```python
from build123d import *

# Parameters (mm, degrees)
F0_W           = 42.3
F0_H           = 42.3
F0_R           = 12
F0_R_2         = 2.5
F0_H_2         = 2
F1_DEPTH       = 5
F2_DEPTH       = 30
F5_D           = 5
F5_DEPTH       = 12.7
F5_TIP         = 1.5021515476
F5_ON_F4_D     = 5
F5_ON_F4_DEPTH = 12.7
F5_ON_F4_TIP   = 1.5021515476


with BuildPart() as f1:
    # F0 (on Top) → F1 (new body)
    with BuildSketch(Plane.XY):
        Polygon((-21.15, 21.15), (21.15, 21.15), (23.15, 21.15), (23.15, 23.15), (-23.15, 23.15), (-23.15, 21.15), align=None)
        Rectangle(F0_W, F0_H)
        with BuildLine():
            ThreePointArc((-15.5, 13.8), (-16.702081528, 16.702081528), (-13.8, 15.5))
            Line((-13.8, 15.5), (13.8, 15.5))
            ThreePointArc((13.8, 15.5), (15.5, 17.2), (17.2, 15.5))
            ThreePointArc((17.2, 15.5), (16.702081528, 14.297918472), (15.5, 13.8))
            Line((15.5, 13.8), (15.5, -13.8))
            ThreePointArc((15.5, -13.8), (16.702081528, -14.297918472), (17.2, -15.5))
            ThreePointArc((17.2, -15.5), (15.5, -17.2), (13.8, -15.5))
            Line((13.8, -15.5), (-13.8, -15.5))
            ThreePointArc((-13.8, -15.5), (-16.702081528, -16.702081528), (-15.5, -13.8))
            Line((-15.5, -13.8), (-15.5, 13.8))
        make_face(mode=Mode.SUBTRACT)
        with BuildLine():
            Line((13.8, 15.5), (-13.8, 15.5))
            ThreePointArc((-13.8, 15.5), (-14.297918472, 14.297918472), (-15.5, 13.8))
            Line((-15.5, 13.8), (-15.5, -13.8))
            ThreePointArc((-15.5, -13.8), (-14.297918472, -14.297918472), (-13.8, -15.5))
            Line((-13.8, -15.5), (13.8, -15.5))
            ThreePointArc((13.8, -15.5), (14.297918472, -14.297918472), (15.5, -13.8))
            Line((15.5, -13.8), (15.5, 13.8))
            ThreePointArc((15.5, 13.8), (14.297918472, 14.297918472), (13.8, 15.5))
        make_face()
        Circle(F0_R, mode=Mode.SUBTRACT)
        Polygon((23.15, 23.15), (23.15, 21.15), (23.15, -23.15), (53.15, -23.15), (53.15, 53.15), (-53.15, 53.15), (-53.15, -23.15), (-23.15, -23.15), (-23.15, 21.15), (-23.15, 23.15), align=None)
        with Locations((-38.15, -8.15)):
            Circle(F0_R_2, mode=Mode.SUBTRACT)
        with Locations((38.15, -8.15)):
            Circle(F0_R_2, mode=Mode.SUBTRACT)
        with Locations((-38.15, 38.15)):
            Circle(F0_R_2, mode=Mode.SUBTRACT)
        with Locations((38.15, 38.15)):
            Circle(F0_R_2, mode=Mode.SUBTRACT)
        Polygon((-21.15, -21.15), (-21.15, 21.15), (-23.15, 21.15), (-23.15, -23.15), (-21.15, -23.15), align=None)
        Polygon((23.15, 21.15), (21.15, 21.15), (21.15, -21.15), (21.15, -23.15), (23.15, -23.15), align=None)
        with Locations((0, -22.15)):
            Rectangle(F0_W, F0_H_2)
    extrude(amount=F1_DEPTH)

    # F0 (on Top) → F2 (join)
    with BuildSketch(Plane.XY):
        Polygon((-21.15, 21.15), (21.15, 21.15), (23.15, 21.15), (23.15, 23.15), (-23.15, 23.15), (-23.15, 21.15), align=None)
        Polygon((23.15, 21.15), (21.15, 21.15), (21.15, -21.15), (21.15, -23.15), (23.15, -23.15), align=None)
    extrude(amount=-F2_DEPTH)

    # F5
    with Locations(Plane.XZ.offset(-21.15)):
        with Locations((0, -15)):
            Hole(F5_D / 2, depth=F5_DEPTH)
            with Locations((0, 0, -(F5_DEPTH + F5_TIP / 2))):  # 118° drill point
                Cone(0, F5_D / 2, F5_TIP, mode=Mode.SUBTRACT)

    # F5 on F4
    with Locations(Plane(origin=(21.15, 0, 0), x_dir=(0, -1, 0), z_dir=(-1, 0, 0))):
        with Locations((0, -15)):
            Hole(F5_ON_F4_D / 2, depth=F5_ON_F4_DEPTH)
            with Locations((0, 0, -(F5_ON_F4_DEPTH + F5_ON_F4_TIP / 2))):  # 118° drill point
                Cone(0, F5_ON_F4_D / 2, F5_ON_F4_TIP, mode=Mode.SUBTRACT)


solid = f1.part
```
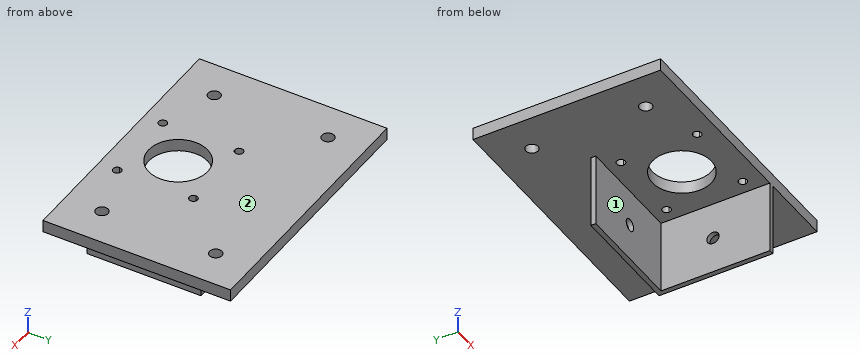
The model under review builds one solid part; all positions refer to its coordinate system, in mm. Face numbers are marked on the shaded views. A direction names the side the tool comes from. Coordinates: 2 decimals unless noted, no trailing zeros. Order: outer loops, then holes, each group sorted by start corner. A loop starts at its lowest first (then second) coordinate and runs counter-clockwise, first axis right, second up. Notation, with made-up numbers: M 74.5,26.5 L 98.5,26.5 A22 cw 98.5,62.5 Z; hole C 85.25,63.25 d2. An arc over 180 degrees is marked long. One line per question, with ' | ' between items.
(1) Add section B-B, the plane y = 0. Write out the cut boundary in (x, z), then the cut area to 4 significant figures.
Geometry results:
outline: M -53.15,0 L -12,0 L -12,5 L -53.15,5 Z; M 12,0 L 21.15,0 L 21.15,-12.5 L 23.15,-12.5 L 23.15,0 L 53.15,0 L 53.15,5 L 12,5 Z; M 21.15,-30 L 23.15,-30 L 23.15,-17.5 L 21.15,-17.5 Z | area: 461.5 mm²
(2) For probe 1 along Y at (x, z) = (-38.15, 2.45); probe 2 along Y at (x, z) = (-15, 1); probe 3 along Z at (x, y) = (0, 22.65), list the stretches that pass through material, from the lowest coordinate up. Write a range as from..to.
Geometry results:
probe 1: y = -23.15..-10.65, -5.65..35.65, 40.65..53.15 | probe 2: y = -23.15..-17.12, -13.88..13.88, 17.12..53.15 | probe 3: z = -30..-17.5, -12.5..5
(3) Insertion check: pin 1 (4 mm diameter, centred on x = 38.15, y = 38.15, fed in from -Z); pin 2 (9 mm diameter, centred on y = -7.5, z = -20.5, fed in from +X); pin 3 (15 mm diameter, centred on x = -7.5, z = -22, fed in from +Y); pin 4 (2 mm diameter, centred on y = -7.5, z = -14.5, fed in from -X). Each pin has a flat end and moves straight along its axis. Give the tip position at first contact, or say it passes through.
Geometry results:
pin 1: passes through | pin 2: stops at x = 23.15 | pin 3: stops at y = 23.15 | pin 4: stops at x = 21.15
(4) Machinability: for the marked faces 1 and 2, which of the approach directions +Z, -Z, +X, -X, +Y, -Y give a long, thin tool a straight path to every point of the face, cutting with its end or side? Answer none if there is none.
Geometry results:
face 1: -Z, -X, -Y | face 2: +Z, +X, -X, +Y, -Y
(5) Add section C-C, the plane z = -23. Write out the cut boundary in (x, y).
Geometry results:
outline: M -23.15,21.15 L 21.15,21.15 L 21.15,-23.15 L 23.15,-23.15 L 23.15,23.15 L -23.15,23.15 Z
(6) Add section A-A, the plane x = -38.15. Write out the cut boundary in (y, z).
Geometry results:
outline: M -23.15,0 L -10.65,0 L -10.65,5 L -23.15,5 Z; M -5.65,0 L 35.65,0 L 35.65,5 L -5.65,5 Z; M 40.65,0 L 53.15,0 L 53.15,5 L 40.65,5 Z
(7) Add section D-D, the plane y = -8.15. Write out the cut boundary in (x, z).
Geometry results:
outline: M -53.15,0 L -40.65,0 L -40.65,5 L -53.15,5 Z; M -35.65,0 L -8.81,0 L -8.81,5 L -35.65,5 Z; M 8.81,0 L 21.15,0 L 21.15,-30 L 23.15,-30 L 23.15,0 L 35.65,0 L 35.65,5 L 8.81,5 Z; M 40.65,0 L 53.15,0 L 53.15,5 L 40.65,5 Z
